```python
from build123d import *

# Parameters (mm, degrees)
F_18_0_1695_DIAMETER_HOLE1_D     = 4.3053
F_18_0_1695_DIAMETER_HOLE1_DEPTH = 11.176
F_18_0_1695_DIAMETER_HOLE1_TIP   = 1.293442612
SKETCH4_R                        = 1.524
CUT_EXTRUDE1_DEPTH               = 11.43
CHAMFER1_SIZE                    = 0.762


with BuildPart() as part:
    # Sketch1 → Revolve1 (revolve)
    with BuildSketch(Plane.XY, mode=Mode.PRIVATE) as revolve1_sk:
        Polygon((0, 0), (0, 16.51), (4.826, 16.51), (5.588, 15.748), (5.588, 6.35), (3.937, 6.35), (3.937, 0), align=None)
    revolve(revolve1_sk.sketch.rotate(Axis((0, 0, 0), (0, -1, 0)), 90), axis=Axis((0, 0, 0), (0, -1, 0)))

    # #18 (0.1695) Diameter Hole1
    with Locations(Plane.XZ):
        with Locations((0, 0)):
            Hole(F_18_0_1695_DIAMETER_HOLE1_D / 2, depth=F_18_0_1695_DIAMETER_HOLE1_DEPTH)
            with Locations((0, 0, -(F_18_0_1695_DIAMETER_HOLE1_DEPTH + F_18_0_1695_DIAMETER_HOLE1_TIP / 2))):  # 118° drill point
                Cone(0, F_18_0_1695_DIAMETER_HOLE1_D / 2, F_18_0_1695_DIAMETER_HOLE1_TIP, mode=Mode.SUBTRACT)

    # Sketch4 → Cut-Extrude1 (cut, symmetric)
    with BuildSketch(Plane(origin=(0, 0, 0), x_dir=(0, 0, -1), z_dir=(1, 0, 0))):
        with Locations((0, 11.176)):
            Circle(SKETCH4_R)
    extrude(amount=CUT_EXTRUDE1_DEPTH, both=True, mode=Mode.SUBTRACT)

    # Chamfer1
    chamfer1_edges = [part.edges().sort_by_distance(p)[0] for p in [
        (0, 0, -3.937),
    ]]
    chamfer(chamfer1_edges, length=CHAMFER1_SIZE)


solid = part.part
```
The listing builds one solid part. Answer for the finished solid, in the listing's coordinates (mm). A direction names the side the tool comes from. Coordinates: 2 decimals unless noted, no trailing zeros. Loops run counter-clockwise (first coordinate to the right, second up) from the corner with the lowest first, then second, coordinate; pieces in that order, holes last. Notation, with made-up numbers: (-1, -2.5) - (42, -2.5) arc R9 cw to (42, 5.5) - close; hole circle Ø7 at (24, 31.25). An arc over 180 degrees is marked (long way). Use a Markdown table: item, result. Add a question column.
1) The mould has two halves that part along X. Classify faces 1 (the cylindrical face through (0.28, 5.666, 2.134)), 2 (the cylindrical face through (4.958, 10.983, 2.579)), 3 (the flat face through (0, 16.51, 0)): released by +X, released by -X, zero draft, split by the parting line, or undercut.
2) The part is cut by section B-B, the plane x = 0. Give the vertices of the cut face in (y, z) (3 decimals), and give its area (3 significant figures).
3) Given pin 1 (1.5 mm diameter, centred on y = 4, z = 2.5, fed in from -X); pin 2 (4 mm diameter, centred on x = 3, y = 10.5, fed in from -Z); pin 3 (6 mm diameter, centred on x = -2, z = -4.5, fed in from -Y); pin 4 (1 mm diameter, centred on x = -3, y = 3, fed in from +Z), each flat-ended and moving along its own axis, determine where each tip first touches the part or whether it passes through.
4) The part is cut by section A-A, the plane z = 0. Give the vertices of the cut face in (x, y) (3 decimals).
5) For faces 4 (the cylindrical face through (0.078, 12.687, 0.198)), 5 (the flat face through (-4, 6.35, 1)), determine the directions among +Z, -Z, +X, -X, +Y, -Y from which every point of the face is accessible in a straight line to the end or side of a thin tool.
6) The part is cut by section C-C, the plane y = 13.5. Give the vertices of the cut face in (x, z).
7) Find the intervals of material crossed by line 1 (X direction, y = 7.5, z = 0); line 2 (Y direction, x = 3.25, z = -3); line 3 (X direction, y = 2.75, z = -1), in increasing order.
Here are the results:
| question | item | result |
|---|---|---|
| 1 | face 1 | undercut |
| 1 | face 2 | split by the parting line |
| 1 | face 3 | zero draft |
| 2 | outline | (0, -3.175) - (0.762, -3.937) - (6.35, -3.937) - (6.35, -5.588) - (15.748, -5.588) - (16.51, -4.826) - (16.51, 4.826) - (15.748, 5.588) - (6.35, 5.588) - (6.35, 3.937) - (0.762, 3.937) - (0, 3.175) - (0, 2.153) - (11.176, 2.153) - (11.588, 1.467) arc R1.524 cw to (11.588, -1.467) - (11.176, -2.153) - (0, -2.153) - close |
| 2 | area | 110 mm^2 |
| 3 | pin 1 | stops at x = -3.53 |
| 3 | pin 2 | stops at z = -5.5 |
| 3 | pin 3 | stops at y = 0 |
| 3 | pin 4 | stops at z = 3.04 |
| 4 | outline | (-5.588, 6.35) - (-3.937, 6.35) - (-3.937, 0.762) - (-3.175, 0) - (-2.153, 0) - (-2.153, 9.652) - (-5.588, 9.652) - close; (-5.588, 12.7) - (5.588, 12.7) - (5.588, 15.748) - (4.826, 16.51) - (-4.826, 16.51) - (-5.588, 15.748) - close; (2.153, 0) - (3.175, 0) - (3.937, 0.762) - (3.937, 6.35) - (5.588, 6.35) - (5.588, 9.652) - (2.153, 9.652) - close |
| 5 | face 4 | +X, -X |
| 5 | face 5 | -Y |
| 6 | outline | circle Ø11.18 at (0, 0) |
| 7 | line 1 | x = -5.59 to -2.15, 2.15 to 5.59 |
| 7 | line 2 | y = 6.35 to 16.51 |
| 7 | line 3 | x = -3.81 to -1.91, 1.91 to 3.81 |
